Can you work these out from the model? Positions are in its coordinate system, mm. A direction names the side the tool comes from. Give positions to 0.01 mm unless a question says otherwise; leave off trailing zeros. Order: outer loops, then holes, each group sorted by start corner. A loop starts at its lowest first (then second) coordinate and runs counter-clockwise, first axis right, second up. Notation, with made-up numbers: M 62.5,44.5 L 91.5,44.5 A35 cw 91.5,78.5 Z; hole C 71,-16 d7. An arc over 180 degrees is marked long. Answer as a JSON object with one key per item and string values.
```python
from build123d import *

# Parameters (mm, degrees)
F0_W           = 16
F0_H           = 24
F1_DEPTH       = 13
F2_W           = 16
F2_H           = 5.8
F3_DEPTH       = 5
F4_DEPTH       = 20
F5_R           = 4.05
F6_DEPTH       = 26.001
F8_D           = 4.4
F8_CBORE_D     = 8.25
F8_CBORE_DEPTH = 2
F9_SIZE        = 1
F11_DEPTH      = 16.001
F12_T1_DEPTH   = 27.2312288127
F12_T3_DEPTH   = 27.2312288127
F12_T5_DEPTH   = 41
F12_T7_DEPTH   = 37.3525491562
F13_R          = 2


# Not quite as in the source:
# - a fillet or chamfer that OpenCascade refuses, or shapes differently, is made with other operations: its cross-section is extruded or revolved along the edge and cut away or added
# - a feature names something its author has since deleted; it is built from what else it names


with BuildPart() as f1:
    # F0 (on Front) → F1 (new body, symmetric)
    with BuildSketch(Plane.XZ):
        Rectangle(F0_W, F0_H)
    extrude(amount=F1_DEPTH, both=True)

    # F2 (on face) → F3 (join)
    with BuildSketch(Plane(origin=(0, 0, -12), x_dir=(1, 0, 0), z_dir=(0, 0, -1))):
        with Locations((0, 3)):
            Rectangle(F2_W, F2_H)
    extrude(amount=F3_DEPTH)

    # F2 (on face) → F4 (join)
    with BuildSketch(Plane(origin=(0, 0, -12), x_dir=(1, 0, 0), z_dir=(0, 0, -1))):
        with Locations((0, -10.1)):
            Rectangle(F2_W, F2_H)
    extrude(amount=F4_DEPTH)

    # F5 (on face) → F6 (cut, through all)
    with BuildSketch(Plane.XZ.offset(13)):
        with Locations((0, 2.95)):
            Circle(F5_R)
    extrude(amount=-F6_DEPTH, mode=Mode.SUBTRACT)

    # F8 (through all)
    with Locations(Plane(origin=(0, 13, 0), x_dir=(-1, 0, 0), z_dir=(0, 1, 0))):
        with Locations((0, -22)):
            CounterBoreHole(F8_D / 2, F8_CBORE_D / 2, F8_CBORE_DEPTH)

    # F9
    f9_edges = [f1.edges().sort_by_distance(p)[0] for p in [
        (0, -5.9, -17),
        (0, -0.1, -17),
    ]]
    chamfer(f9_edges, length=F9_SIZE)

    # F10 (on face) → F11 (cut, through all)
    with BuildSketch(Plane.YZ.offset(8)):
        with BuildLine():
            Line((-13, 12), (-0.5, 12))
            ThreePointArc((-0.5, 12), (-21.8388347648, 20.8388347648), (-13, -0.5))
            Line((-13, -0.5), (-13, 12))
        make_face()
        with BuildLine():
            ThreePointArc((-13, -0.5), (-4.1611652352, 3.1611652352), (-0.5, 12))
            Line((-0.5, 12), (-13, 12))
            Line((-13, 12), (-13, -0.5))
        make_face()
    extrude(amount=-F11_DEPTH, mode=Mode.SUBTRACT)

    # F12: fillet of radius 5 on 5 edges, made by hand

    # F12_s2 → F12_t1 (cut)
    with BuildSketch(Plane.YZ.offset(-8.5549542346)):
        with BuildLine():
            ThreePointArc((-9.4285714286, 0.0210644063), (-12.0089186287, -1.7824383079), (-13, -4.7705098312))
            Line((-13, -4.7705098312), (-13, -0.5))
            ThreePointArc((-13, -0.5), (-11.1953802231, -0.369047961), (-9.4285714286, 0.0210644063))
        make_face()
    extrude(amount=F12_T1_DEPTH, mode=Mode.SUBTRACT)

    # F12_s4 → F12_t3 (cut)
    with BuildSketch(Plane.YZ.offset(-18.6762745781)):
        with BuildLine():
            ThreePointArc((-9.4285714286, 0.0210644063), (-12.0089186287, -1.7824383079), (-13, -4.7705098312))
            Line((-13, -4.7705098312), (-13, -0.5))
            ThreePointArc((-13, -0.5), (-11.1953802231, -0.369047961), (-9.4285714286, 0.0210644063))
        make_face()
    extrude(amount=F12_T3_DEPTH, mode=Mode.SUBTRACT)

    # F12_s6 → F12_t5 (cut)
    with BuildSketch(Plane.YZ.offset(-20.5)):
        with BuildLine():
            ThreePointArc((8, -32), (11.5355339059, -30.5355339059), (13, -27))
            Line((13, -27), (13, -32))
            Line((13, -32), (8, -32))
        make_face()
        with BuildLine():
            ThreePointArc((13, 7), (11.5355339059, 10.5355339059), (8, 12))
            Line((8, 12), (13, 12))
            Line((13, 12), (13, 7))
        make_face()
    extrude(amount=F12_T5_DEPTH, mode=Mode.SUBTRACT)

    # F12_s8 → F12_t7 (cut)
    with BuildSketch(Plane.YZ.offset(-18.6762745781)):
        with BuildLine():
            ThreePointArc((3.7705098312, 12), (0.7824383079, 11.0089186287), (-1.0210644063, 8.4285714286))
            ThreePointArc((-1.0210644063, 8.4285714286), (-0.630952039, 10.1953802231), (-0.5, 12))
            Line((-0.5, 12), (3.7705098312, 12))
        make_face()
    extrude(amount=F12_T7_DEPTH, mode=Mode.SUBTRACT)

    # F13
    f13_edges = [f1.edges().sort_by_distance(p)[0] for p in [
        (0, -13, -12),
    ]]
    fillet(f13_edges, radius=F13_R)


solid = f1.part
```
1) I'm going to push flat-ended pins straight in: pin 1 Ø3 at (x, y) = (-1, -1.5) entering from +Z; pin 2 Ø5 at (x, y) = (-6, -2.5) entering from -Z; pin 3 Ø8 at (x, z) = (-1, -26.5) entering from -Y. Where does each tip first touch, or does it pass through?
Results found:
{"pin 1": "stops at z = 10.28", "pin 2": "stops at z = -17", "pin 3": "stops at y = 7.2"}
2) I want a section at D-D on z = 2. Write out the boundary of the cut face in (x, y), and give its area (3 significant figures).
Results found:
{"outline": "M -8,-5.5 L -3.94,-5.5 L -3.94,13 L -8,13 Z; M 3.94,-5.5 L 8,-5.5 L 8,13 L 3.94,13 Z", "area": "150 mm²"}
3) I need wall thicknesses on L1, parallel to Z at x = 0, y = 7.25; L2, parallel to Z at x = 1, y = 7.75; L3, parallel to Y at x = 2.75, z = -16. Which ranges of each line are inside material? Lowest first, please.
Results found:
{"L1": "z = -32 to -24.2, -19.8 to -1.1, 7 to 12", "L2": "z = -32 to -23.96, -20.04 to -0.97, 6.87 to 12", "L3": "y = -5.9 to -0.1, 7.2 to 13"}
4) I want a section at A-A on z = -22. Write out the boundary of the cut face in (x, y) (3 decimals).
Results found:
{"outline": "M -8,7.2 L -2.2,7.2 L -2.2,11 L -4.125,11 L -4.125,13 L -8,13 Z; M 2.2,7.2 L 8,7.2 L 8,13 L 4.125,13 L 4.125,11 L 2.2,11 Z"}
5) Thinking about a two-plate mould opening in Z: for faces 4 (the face through (-0.9, 3.3, -1)), 5 (the face through (0, 12, 10)), 6 (the face through (0, 13, -10)), which applies, pulls with the +Z half, pulls with the -Z half, needs draft (parallel to the pull), parting line crosses it, or undercut?
Results found:
{"face 4": "undercut", "face 5": "pulls with the +Z half", "face 6": "needs draft"}
6) For faces 1 (the face through (-0.1, -0.6, -16.5)), 2 (the face through (0, -8, -12)), 3 (the face through (1, 12, -18)), which set-ups out of +Z, -Z, +X, -X, +Y, -Y let a thin tool reach every point of the face, with its end or its side?
Results found:
{"face 1": "-Z, +X, -X", "face 2": "-Z, +X, -X, -Y", "face 3": "+Y"}
7) I want a section at B-B on x = 5. Write out the boundary of the cut face in (y, z).
Results found:
{"outline": "M -13,-10 A2 ccw -11,-12 L -5.9,-12 L -5.9,-16 L -4.9,-17 L -1.1,-17 L -0.1,-16 L -0.1,-12 L 7.2,-12 L 7.2,-32 L 8,-32 A5 ccw 13,-27 L 13,7 A5 ccw 8,12 L 3.77,12 A5 ccw -1.02,8.43 A12.5 cw -9.43,0.02 A5 ccw -13,-4.77 Z"}
8) I want a section at C-C on x = 0.75. Count the separate pieces of the cut face and the enclosed holes in it, and give its area (3 significant figures).
Results found:
{"separate pieces": "3", "enclosed holes": "0", "area": "451 mm²"}
